Geometry check sheet. Reference: the model listing, model coordinates, mm. Face numbers are marked on the shaded views. A direction names the side the tool comes from. Coordinates: 2 decimals unless noted, no trailing zeros. Write each loop counter-clockwise with the first axis right and the second up, starting at its lowest first coordinate (ties: lowest second). Pieces come first, ordered by that corner, then holes. Notation, with made-up numbers: M 56.25,-4 L 108.25,-4 A22 cw 108.25,12 Z; hole C -20,-28 d5. An arc over 180 degrees is marked long. Put each result on its own line as item: value. Start each with the question number.
1) Scan lines: line 1 along Y through (x, z) = (-8, 84); line 2 along X through (y, z) = (15.25, 54); line 3 along Z through (x, y) = (8.25, 9). Record each from-to range of solid material in increasing order.
2) Gauge pin test, flat ends, axial feed: pin 1 (3.5 mm diameter, centred on x = 0, z = -2.5, fed in from +Y); pin 2 (0.6 mm diameter, centred on y = 16, z = 71.5, fed in from -X); pin 3 (3.5 mm diameter, centred on y = 11.5, z = -3, fed in from +X); pin 4 (1.5 mm diameter, centred on x = 1, y = 4.5, fed in from +Z). Record the tip position at first contact, or that the pin passes through.
3) Mould release check, pull along Y, two halves, no side actions. Record for the marked faces 3, 4 and 5: released by +Y, released by -Y, zero draft, split by the parting line, or undercut.
4) Set-up check for the marked faces 1 and 2: record each of +Z, -Z, +X, -X, +Y, -Y from which the full face is reachable in a straight line by a thin tool's end or side.
5) Cross-section at D-D on x = -2.5. Count the separate pieces of the cut face and the enclosed holes in it, plus the area to 3 significant figures.
6) Cross-section at B-B on z = 42. Record the cut outline in (x, y).
from build123d import *

# Parameters (mm, degrees)
F0_W      = 30
F0_H      = 20
F1_DEPTH  = 90
F2_R      = 3
F3_W      = 26
F3_H      = 16
F4_DEPTH  = 100
F5_W      = 27
F5_H      = 17
F6_DEPTH  = 4.5
F7_DEPTH  = 5
F8_R      = 3.0778907451
F8_W      = 2
F8_H      = 2
F9_DEPTH  = 2
F10_W     = 7
F10_H     = 7
F11_DEPTH = 0.5
F12_W     = 26
F12_H     = 8.5281978436
F13_DEPTH = 2
F14_W     = 14
F14_H     = 8.5281978436
F15_DEPTH = 2
F16_W     = 24
F16_H     = 8.5281978436
F17_DEPTH = 2
F18_W     = 12
F18_H     = 8.5281978436
F19_DEPTH = 2
F20_R     = 1.99999


# Not quite as in the source:
# - a fillet or chamfer is up to 0.001 mm smaller than in the source, because OpenCascade refuses the exact size


with BuildPart() as f1:
    # F0 (on Top) → F1 (new body)
    with BuildSketch(Plane.XY):
        with Locations((-4.6270154417, 7.9813233296)):
            Rectangle(F0_W, F0_H)
    extrude(amount=F1_DEPTH)

    # F2
    f2_edges = [f1.edges().sort_by_distance(p)[0] for p in [
        (-19.627015, -2.018677, 45),
        (-19.627015, 17.981323, 45),
        (10.372985, -2.018677, 45),
        (10.372985, 17.981323, 45),
    ]]
    fillet(f2_edges, radius=F2_R)

    # F3 (on face) → F4 (cut)
    with BuildSketch(Plane.XY.offset(90)):
        with Locations((-4.6270154417, 7.9813233296)):
            Rectangle(F3_W, F3_H)
    extrude(amount=-F4_DEPTH, mode=Mode.SUBTRACT)

    # F5 (on face) → F6 (join)
    with BuildSketch(Plane(origin=(0, 0, 0), x_dir=(1, 0, 0), z_dir=(0, 0, -1))):
        with Locations((-4.6270154417, -7.9813233296)):
            Rectangle(F5_W, F5_H)
    extrude(amount=F6_DEPTH)

    # F7 (cut): a face of the model
    f7_faces = [f1.faces().sort_by_distance(p)[0] for p in [
        (-4.6270154417, 7.9813233296, 0),
    ]]
    extrude(f7_faces, amount=-F7_DEPTH, mode=Mode.SUBTRACT)

    # F8 (on face) → F9 (cut)
    with BuildSketch(Plane(origin=(0, 17.9813233296, 0), x_dir=(-1, 0, 0), z_dir=(0, 1, 0))):
        with Locations((4.6270154417, 71.1657330394)):
            Circle(F8_R)
        with Locations((4.6270154417, 82.6890671849)):
            Rectangle(F8_W, F8_H)
    extrude(amount=-F9_DEPTH, mode=Mode.SUBTRACT)

    # F10 (on face) → F11 (cut)
    with BuildSketch(Plane.XZ.offset(-15.9813233296)):
        with Locations((-4.6607098193, 71.1224186855)):
            Rectangle(F10_W, F10_H)
    extrude(amount=-F11_DEPTH, mode=Mode.SUBTRACT)

    # F12 (on face) → F13 (join)
    with BuildSketch(Plane.XZ.offset(-15.9813233296)):
        with Locations((-4.6270154417, -0.2359010782)):
            Rectangle(F12_W, F12_H)
    extrude(amount=F13_DEPTH)

    # F14 (on face) → F15 (join)
    with BuildSketch(Plane(origin=(8.3729845583, 0, 0), x_dir=(0, -1, 0), z_dir=(-1, 0, 0))):
        with Locations((-6.9813233296, -0.2359010782)):
            Rectangle(F14_W, F14_H)
    extrude(amount=F15_DEPTH)

    # F16 (on face) → F17 (join)
    with BuildSketch(Plane(origin=(0, -0.0186766704, 0), x_dir=(-1, 0, 0), z_dir=(0, 1, 0))):
        with Locations((5.6270154417, -0.2359010782)):
            Rectangle(F16_W, F16_H)
    extrude(amount=F17_DEPTH)

    # F18 (on face) → F19 (join)
    with BuildSketch(Plane.YZ.offset(-17.6270154417)):
        with Locations((7.9813233296, -0.2359010782)):
            Rectangle(F18_W, F18_H)
    extrude(amount=F19_DEPTH)

    # F20 (radius 2 in the source; OpenCascade refuses exactly that, so slightly less here)
    f20_edges = [f1.edges().sort_by_distance(p)[0] for p in [
        (-15.627015, 7.981323, 4.028198),
        (-4.627015, 1.981323, 4.028198),
        (6.372985, 7.981323, 4.028198),
        (-4.627015, 13.981323, 4.028198),
    ]]
    fillet(f20_edges, radius=F20_R)


solid = f1.part
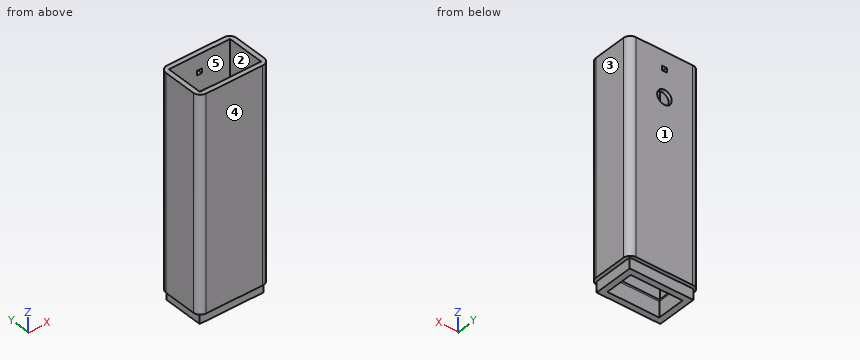
Answer key:
1. line 1: y = -2.02 to -0.02, 15.98 to 17.98
1. line 2: x = -19.61 to -17.63, 8.37 to 10.36
1. line 3: z = -4.5 to 4.02
2. pin 1: stops at y = 16.48
2. pin 2: stops at x = -19.54
2. pin 3: stops at x = 8.87
2. pin 4: passes through
3. face 3: zero draft
3. face 4: released by -Y
3. face 5: undercut
4. face 1: +Z, -Z, +X, -X, +Y
4. face 2: +Z
5. separate pieces: 3
5. enclosed holes: 0
5. area: 387 mm²
6. outline: M -19.63,0.98 A3 ccw -16.63,-2.02 L 7.37,-2.02 A3 ccw 10.37,0.98 L 10.37,14.98 A3 ccw 7.37,17.98 L -16.63,17.98 A3 ccw -19.63,14.98 Z; hole M -17.63,-0.02 L 8.37,-0.02 L 8.37,15.98 L -17.63,15.98 Z
